For this review, take the finished solid that the model builds, in its own axes (mm). Coordinates: 2 decimals unless noted, no trailing zeros. Order: outer loops, then holes, each group sorted by start corner. A loop starts at its lowest first (then second) coordinate and runs counter-clockwise, first axis right, second up. Notation, with made-up numbers: (63.5, 37.5) -> (113.5, 37.5) arc R34 cw to (113.5, 68.5) -> close; hole circle Ø9 at (76.5, 81.25). An arc over 180 degrees is marked (long way). Write item = value, one per line. Start each with the question number.
1) Consider section A-A on x = 25.4. Give the boundary of the cut face in (y, z), and give its area (3 significant figures).
2) Consider section B-B on z = -74. Give the boundary of the cut face in (x, y), and give its area (3 significant figures).
3) Wall thickness on probe 1 along X at (y, z) = (2.35, -33.5); probe 2 along X at (y, z) = (3.05, -70.5); probe 3 along X at (y, z) = (2.6, -73): over which ranges is each line inside the solid? List them lowest first. Write a range as [from, to].
4) Consider section D-D on x = 5.5. Give the boundary of the cut face in (y, z).
5) Insertion check: pin 1 Ø1.5 at (y, z) = (4.5, -77.5) entering from -X; pin 2 Ø19 at (x, z) = (25.4, -77.25) entering from +Y; pin 3 Ø5 at (x, z) = (12, -56.5) entering from +Y. Each pin has a flat end and moves straight along its axis. Give the tip position at first contact, or say it passes through.
from build123d import *

# Parameters (mm, degrees)
SKETCH1_W           = 50.8
SKETCH1_H           = 101.6
BOSS_EXTRUDE1_DEPTH = 76.962
CUT_EXTRUDE1_DEPTH  = 138.209144899
SKETCH6_R           = 8.255
CUT_EXTRUDE2_DEPTH  = 114.705788771
CUT_EXTRUDE3_DEPTH  = 114.705788909


with BuildPart() as part:
    # Sketch1 → Boss-Extrude1 (new body)
    with BuildSketch(Plane(origin=(0, 0, 0), x_dir=(1, 0, 0), z_dir=(0, 1, 0))):
        with Locations((25.4, 50.8)):
            Rectangle(SKETCH1_W, SKETCH1_H)
    extrude(amount=BOSS_EXTRUDE1_DEPTH)

    # Sketch2 → Cut-Extrude1 (cut, through all)
    with BuildSketch(Plane(origin=(50.8, 0, 0), x_dir=(0, 0, -1), z_dir=(1, 0, 0))):
        with BuildLine():
            ThreePointArc((0, 0), (50.8, 5.08), (101.6, 0))
            Line((101.6, 0), (101.6, 76.962))
            Line((101.6, 76.962), (0, 76.962))
            Line((0, 76.962), (0, 0))
        make_face()
    extrude(amount=-CUT_EXTRUDE1_DEPTH, mode=Mode.SUBTRACT)

    # Sketch6 → Cut-Extrude2 (cut, through all)
    with BuildSketch(Plane.XZ):
        with Locations(Location((25.4, -77.250605012, 0), (0, 0, 270))):
            Circle(SKETCH6_R)
    extrude(amount=-CUT_EXTRUDE2_DEPTH, mode=Mode.SUBTRACT)

    # Sketch5 → Cut-Extrude3 (cut, through all)
    with BuildSketch(Plane.XZ):
        with BuildLine():
            Line((21.377665877, -34.538594366), (21.377665877, -38.875260441))
            ThreePointArc((21.377665877, -38.875260441), (18.798754023, -41.454172295), (16.219842169, -38.875260441))
            Line((16.219842169, -38.875260441), (16.219842169, -34.538594366))
            ThreePointArc((16.219842169, -34.538594366), (18.798754023, -31.959682512), (21.377665877, -34.538594366))
        make_face()
        with BuildLine():
            Line((34.582973156, -34.538594366), (34.582973156, -38.875260441))
            ThreePointArc((34.582973156, -38.875260441), (32.004061302, -41.454172295), (29.425149448, -38.875260441))
            Line((29.425149448, -38.875260441), (29.425149448, -34.538594366))
            ThreePointArc((29.425149448, -34.538594366), (32.004061302, -31.959682512), (34.582973156, -34.538594366))
        make_face()
        with BuildLine():
            Line((22.354769429, -53.669734582), (28.407840078, -53.669734582))
            ThreePointArc((28.407840078, -53.669734582), (31.442451437, -56.704345941), (28.407840078, -59.7389573))
            Line((28.407840078, -59.7389573), (22.354769429, -59.7389573))
            ThreePointArc((22.354769429, -59.7389573), (19.32015807, -56.704345941), (22.354769429, -53.669734582))
        make_face()
    extrude(amount=-CUT_EXTRUDE3_DEPTH, mode=Mode.SUBTRACT)


solid = part.part
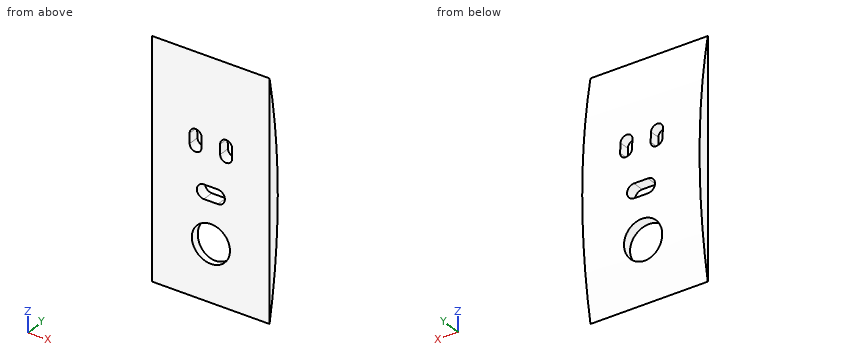
Answer sheet:
q1.outline = (0, -101.6) arc R256.54 ccw to (2.72, -85.51) -> (0, -85.51) -> close; (0, -69) -> (4.43, -69) arc R256.54 ccw to (4.92, -59.74) -> (0, -59.74) -> close; (0, -53.67) -> (5.06, -53.67) arc R256.54 ccw to (0, 0) -> close
q1.area = 254 mm2
q2.outline = (0, 0) -> (17.81, 0) -> (17.81, 4.03) -> (0, 4.03) -> close; (32.99, 0) -> (50.8, 0) -> (50.8, 4.03) -> (32.99, 4.03) -> close
q2.area = 144 mm2
q3.probe_1 = [0, 16.44], [21.16, 29.64], [34.36, 50.8]
q3.probe_2 = [0, 20.65], [30.15, 50.8]
q3.probe_3 = [0, 18.32], [32.48, 50.8]
q4.outline = (0, -101.6) arc R256.54 ccw to (0, 0) -> close
q5.pin_1 = through
q5.pin_2 = 4.52
q5.pin_3 = 5.06
